Can you work these out from the model? Positions are in its coordinate system, mm. A direction names the side the tool comes from. Round coordinates to 2 decimals unless told otherwise and drop trailing zeros. Loops run counter-clockwise (first coordinate to the right, second up) from the corner with the lowest first, then second, coordinate; pieces in that order, holes last. Notation, with made-up numbers: (76.25, 77.5) -> (130.25, 77.5) arc R28 ccw to (130.25, 112.5) -> close; hole circle Ø11 at (-10, 3.25). An arc over 180 degrees is marked (long way). Write each question's results on one line, items separated by ' | '.
from build123d import *

# Parameters (mm, degrees)
F2_W     = 20
F2_H     = 10
F3_DEPTH = 2
F4_W     = 10
F4_H     = 10
F5_DEPTH = 25


with BuildPart() as f1:
    # F0 (on Front) → F1 (revolve)
    with BuildSketch(Plane.XZ):
        Polygon((0, 13.617994), (0, 28.617994), (-30, 28.617994), (-30, 23.617994), (-25, 23.617994), (-25, 13.617994), align=None)
    revolve(axis=Axis((0, 0, -2.582015), (0, 0, -1)))

    # F2 (on face) → F3 (cut)
    with BuildSketch(Plane.XY.offset(28.617994)):
        Rectangle(F2_W, F2_H)
    extrude(amount=-F3_DEPTH, mode=Mode.SUBTRACT)

    # F4 (on face) → F5 (cut)
    with BuildSketch(Plane.XY.offset(26.617994)):
        Rectangle(F4_W, F4_H)
    extrude(amount=-F5_DEPTH, mode=Mode.SUBTRACT)


solid = f1.part
1. If we section it at C-C (z = 22.75): List the corners of the cut face in (x, y) for me, then the cut area to 3 significant figures.
Final values:
outline: circle Ø50 at (0, 0); hole (-5, -5) -> (5, -5) -> (5, 5) -> (-5, 5) -> close | area: 1,860 mm2
2. If we section it at D-D (y = 9): List the corners of the cut face in (x, z) for me, then the cut area to 3 significant figures.
Final values:
outline: (-28.62, 23.62) -> (-23.32, 23.62) -> (-23.32, 13.62) -> (23.32, 13.62) -> (23.32, 23.62) -> (28.62, 23.62) -> (28.62, 28.62) -> (-28.62, 28.62) -> close | area: 753 mm2
3. We'd pull the mould along X, two halves only. Please class faces 1 (the face through (0, 5, 21)), 2 (the face through (0, -6, 28.618)), 3 (the face through (-23.846, 7.509, 18.548)), 4 (the face through (-5, 0, 20)): pulls with the +X half, pulls with the -X half, needs draft (parallel to the pull), parting line crosses it, or undercut.
Final values:
face 1: undercut | face 2: needs draft | face 3: parting line crosses it | face 4: undercut
4. On a 3-axis mill with a long thin cutter (end or side, diameter ignored), from which of +Z, -Z, +X, -X, +Y, -Y can I reach the whole of each face in a straight line? I mean faces 5 (the face through (7, 25, 23.618)), 6 (the face through (0.3, -5.2, 13.618)), 7 (the face through (7, 0, 26.618)), 8 (the face through (5, 0, 20)). Say none if no direction works.
Final values:
face 5: -Z | face 6: -Z, +X, -X, +Y, -Y | face 7: +Z | face 8: +Z, -Z
5. Will these pins go through, and if not, where does the flat tip stop? pin 1 (6 mm diameter, centred on x = 5.5, z = 15.5, fed in from -Y); pin 2 (0.6 mm diameter, centred on y = 1.5, z = 28, fed in from -X); pin 3 (1 mm diameter, centred on y = -1.5, z = 27.5, fed in from +X).
Final values:
pin 1: y = -24.87 | pin 2: x = -29.98 | pin 3: x = 29.98
6. If we section it at A-A (y = 0): List the corners of the cut face in (x, z) for me, then the cut area to 3 significant figures.
Final values:
outline: (-30, 23.62) -> (-25, 23.62) -> (-25, 13.62) -> (-5, 13.62) -> (-5, 26.62) -> (-10, 26.62) -> (-10, 28.62) -> (-30, 28.62) -> close; (5, 13.62) -> (25, 13.62) -> (25, 23.62) -> (30, 23.62) -> (30, 28.62) -> (10, 28.62) -> (10, 26.62) -> (5, 26.62) -> close | area: 630 mm2
7. If we section it at B-B (x = 0): List the corners of the cut face in (y, z) for me.
Final values:
outline: (-30, 23.62) -> (-25, 23.62) -> (-25, 13.62) -> (-5, 13.62) -> (-5, 28.62) -> (-30, 28.62) -> close; (5, 13.62) -> (25, 13.62) -> (25, 23.62) -> (30, 23.62) -> (30, 28.62) -> (5, 28.62) -> close
8. Please list where these lines run through material, in increasing order: line 1 (Z direction, x = 24, y = 14); line 2 (X direction, y = 1, z = 20.75); line 3 (Y direction, x = 8.5, z = 20.5). Write a range as from..to.
Final values:
line 1: 23.62..28.62 | line 2: -24.98..-5, 5..24.98 | line 3: -23.51..23.51
